Model file for the job. Use its own axes, mm. A direction names the side the tool comes from. Coordinates: 2 decimals unless noted, no trailing zeros.
from build123d import *

# Parameters (mm, degrees)
F0_W     = 914.4
F0_H     = 457.2
F1_DEPTH = 1644.65
F2_W     = 838.2
F2_H     = 307.975
F2_W_2   = 155.575
F2_H_2   = 38.1
F2_H_3   = 306.705
F2_H_4   = 322.58
F3_DEPTH = 1.905
F2_H_5   = 1.27
F4_DEPTH = 25.4
F5_DEPTH = 12.7


with BuildPart() as f1:
    # F0 (on Top) → F1 (new body)
    with BuildSketch(Plane.XY):
        with Locations((457.2, 228.6)):
            Rectangle(F0_W, F0_H)
    extrude(amount=F1_DEPTH)

    # F2 (on face) → F3 (cut)
    with BuildSketch(Plane.XZ):
        with Locations((457.2, 192.0875)):
            Rectangle(F2_W, F2_H)
        with Locations((457.2, 238.125)):
            Rectangle(F2_W_2, F2_H_2, mode=Mode.SUBTRACT)
        with Locations((457.2, 500.6975)):
            Rectangle(F2_W, F2_H_3)
        with Locations((457.2, 546.1)):
            Rectangle(F2_W_2, F2_H_2, mode=Mode.SUBTRACT)
        with Locations((457.2, 808.6725)):
            Rectangle(F2_W, F2_H_3)
        with Locations((457.2, 854.075)):
            Rectangle(F2_W_2, F2_H_2, mode=Mode.SUBTRACT)
        with Locations((457.2, 1128.7125)):
            Rectangle(F2_W, F2_H)
        with Locations((457.2, 1174.75)):
            Rectangle(F2_W_2, F2_H_2, mode=Mode.SUBTRACT)
        with Locations((457.2, 1445.26)):
            Rectangle(F2_W, F2_H_4)
        with Locations((457.2, 1317.625)):
            Rectangle(F2_W_2, F2_H_2, mode=Mode.SUBTRACT)
    extrude(amount=-F3_DEPTH, mode=Mode.SUBTRACT)

    # F2 (on face) → F4 (cut)
    with BuildSketch(Plane.XZ):
        with Locations((457.2, 346.71)):
            Rectangle(F2_W, F2_H_5)
        with Locations((457.2, 654.685)):
            Rectangle(F2_W, F2_H_5)
        with Locations((457.2, 1283.335)):
            Rectangle(F2_W, F2_H_5)
    extrude(amount=-F4_DEPTH, mode=Mode.SUBTRACT)

    # F2 (on face) → F5 (cut)
    with BuildSketch(Plane.XZ):
        with Locations((457.2, 1317.625)):
            Rectangle(F2_W_2, F2_H_2)
        with Locations((457.2, 1174.75)):
            Rectangle(F2_W_2, F2_H_2)
        with Locations((457.2, 854.075)):
            Rectangle(F2_W_2, F2_H_2)
        with Locations((457.2, 546.1)):
            Rectangle(F2_W_2, F2_H_2)
        with Locations((457.2, 238.125)):
            Rectangle(F2_W_2, F2_H_2)
    extrude(amount=-F5_DEPTH, mode=Mode.SUBTRACT)


solid = f1.part
Q1. Drill centre lines: line 1 (Z direction, x = 346, y = 24.5) (3 decimals); line 2 (Y direction, x = 436, z = 172) (3 decimals). Where is each one in solid material? Low to high.
Answers:
line 1: z = 0 to 346.075, 347.345 to 654.05, 655.32 to 1282.7, 1283.97 to 1644.65
line 2: y = 1.905 to 457.2
Q2. Mould opens along Z. For faces 3 (the flat face through (451, 232, 0)), 4 (the flat face through (456, 12.7, 1175)), 5 (the flat face through (914.4, 225, 811)) say: +Z half, -Z half, draft (parallel to the pull), parting line (faces both ways), or undercut.
Answers:
face 3: -Z half
face 4: undercut
face 5: draft
Q3. Flat gauge pins, fed straight in: P1, Ø6, axis at x = 803.5, y = 364.5, coming from the -Z side; P2, Ø12, axis at x = 211.5, z = 232.5, coming from the -Y side (3 decimals). Where does each tip first touch, or does it go through?
Answers:
P1: stops at z = 0
P2: stops at y = 1.905
Q4. Which spindle directions (+Z, -Z, +X, -X, +Y, -Y) get a long thin tool onto all of the face, cutting with end or side? Do faces 1 (the flat face through (15, 0, 818)), 2 (the flat face through (451, 1.905, 1448)). Say none if no direction does.
Answers:
face 1: +Z, -Z, +X, -X, -Y
face 2: -Y
